```python
from build123d import *

# Parameters (mm, degrees)
ESQUISSE1_W      = 350
ESQUISSE1_H      = 350
EXTRUSION1_DEPTH = 350
ESQUISSE2_R      = 10
EXTRUSION2_DEPTH = 80
ESQUISSE3_W      = 80
ESQUISSE3_H      = 80
EXTRUSION3_DEPTH = 80


with BuildPart() as part:
    # Esquisse1 → Extrusion1 (new body)
    with BuildSketch(Plane(origin=(0, 0, 0), x_dir=(1, 0, 0), z_dir=(0, 1, 0))):
        with Locations((175, 175)):
            Rectangle(ESQUISSE1_W, ESQUISSE1_H)
    extrude(amount=EXTRUSION1_DEPTH)

    # Esquisse2 → Extrusion2 (add)
    with BuildSketch(Plane(origin=(0, 350, 0), x_dir=(1, 0, 0), z_dir=(0, 1, 0))):
        with Locations((175, 175)):
            Circle(ESQUISSE2_R)
    extrude(amount=EXTRUSION2_DEPTH)

    # Esquisse3 → Extrusion3 (add)
    with BuildSketch(Plane(origin=(0, 430, 0), x_dir=(1, 0, 0), z_dir=(0, 1, 0))):
        with Locations((175, 175)):
            Rectangle(ESQUISSE3_W, ESQUISSE3_H)
    extrude(amount=EXTRUSION3_DEPTH)


solid = part.part
```
Part model, mm, in its own coordinate system. A direction names the side the tool comes from. Round coordinates to 2 decimals unless told otherwise and drop trailing zeros. Write each loop counter-clockwise with the first axis right and the second up, starting at its lowest first coordinate (ties: lowest second). Pieces come first, ordered by that corner, then holes. Notation, with made-up numbers: (81, 48) -> (106, 48) arc R19 cw to (106, 71) -> close; hole circle Ø11 at (22.25, -8.75). An arc over 180 degrees is marked (long way). Return JSON: item names as keys, results as strings. Group by question number.
Q1. Saw through at C-C on y = 379. Write the cut outline in (x, z).
Q2. Saw through at D-D on x = 40. Write the cut outline in (y, z).
Q3. Pin check, flat tip, straight feed: pin 1 (24 mm diameter, centred on x = 183, y = 475.5, fed in from +Z). Stop position of the tip, or through.
Q4. Mould opens along Y. For faces 1 (the flat face through (173, 173, -350)), 2 (the flat face through (173, 0, -177)), 3 (the cylindrical face through (184.237, 389.44, -171.17)) say: pulls with the +Y half, pulls with the -Y half, needs draft (parallel to the pull), parting line crosses it, or undercut.
Q5. Saw through at B-B on x = 175. Write the cut outline in (y, z), plus the area to 4 significant figures.
Q6. Which spindle directions (+Z, -Z, +X, -X, +Y, -Y) get a long thin tool onto all of the face, cutting with end or side? Do faces 4 (the flat face through (174, 469, -135)), 5 (the flat face through (215, 469, -174)), 6 (the flat face through (166, 430, -167)), 7 (the flat face through (135, 469, -174)), 8 (the flat face through (174, 469, -215)). Say none if no direction does.
Q7. Saw through at A-A on z = -175. Write the cut outline in (x, y).
Q8. Probe L1, parallel to Y at x = 210, z = -40; L2, parallel to X at y = 445.5, z = -170. List the from-to ranges inside material, lowest first. Write a range as [from, to].
Answer:
{
 "1": {"outline": "circle Ø20 at (175, -175)"},
 "2": {"outline": "(0, -350) -> (350, -350) -> (350, 0) -> (0, 0) -> close"},
 "3": {"pin 1": "z = -135"},
 "4": {"face 1": "needs draft", "face 2": "pulls with the -Y half", "face 3": "undercut"},
 "5": {"outline": "(0, -350) -> (350, -350) -> (350, -185) -> (430, -185) -> (430, -215) -> (510, -215) -> (510, -135) -> (430, -135) -> (430, -165) -> (350, -165) -> (350, 0) -> (0, 0) -> close", "area": "130,500 mm2"},
 "6": {"face 4": "+Z, +X, -X, +Y", "face 5": "+Z, -Z, +X, +Y", "face 6": "none", "face 7": "+Z, -Z, -X, +Y", "face 8": "-Z, +X, -X, +Y"},
 "7": {"outline": "(0, 0) -> (350, 0) -> (350, 350) -> (185, 350) -> (185, 430) -> (215, 430) -> (215, 510) -> (135, 510) -> (135, 430) -> (165, 430) -> (165, 350) -> (0, 350) -> close"},
 "8": {"L1": "[0, 350]", "L2": "[135, 215]"}
}
